CAD build for the part. Positions are in the model's coordinates, mm. A direction names the side the tool comes from. Give positions to 0.01 mm unless a question says otherwise; leave off trailing zeros. Order: outer loops, then holes, each group sorted by start corner. A loop starts at its lowest first (then second) coordinate and runs counter-clockwise, first axis right, second up.
from build123d import *

# Parameters (mm, degrees)
F0_W      = 45
F0_H      = 30
F1_DEPTH  = 3
F2_R      = 5
F3_DEPTH  = 1
F4_R      = 2.5
F5_DEPTH  = 2
F6_W      = 10
F6_H      = 30
F7_DEPTH  = 80
F9_DEPTH  = 2.5
F10_R     = 8.5
F11_DEPTH = 10
F12_R     = 10
F13_R     = 10
F14_R     = 5
F15_R     = 5


with BuildPart() as f1:
    # F0 (on Top) → F1 (new body)
    with BuildSketch(Plane.XY):
        Rectangle(F0_W, F0_H)
    extrude(amount=F1_DEPTH)

    # F2 (on face) → F3 (cut)
    with BuildSketch(Plane.XY.offset(3)):
        with Locations((-11.25, 0)):
            Circle(F2_R)
    extrude(amount=-F3_DEPTH, mode=Mode.SUBTRACT)

    # F4 (on face) → F5 (cut, through all)
    with BuildSketch(Plane.XY.offset(2)):
        with Locations((-11.25, 0)):
            Circle(F4_R)
    extrude(amount=-F5_DEPTH, mode=Mode.SUBTRACT)

    # F6 (on face) → F7 (join)
    with BuildSketch(Plane.XY.offset(3)):
        with Locations((17.5, 0)):
            Rectangle(F6_W, F6_H)
    extrude(amount=F7_DEPTH)

    # F8 (on Front) → F9 (join, symmetric)
    with BuildSketch(Plane.XZ):
        Polygon((12.5, 38), (-2.5, 3), (12.5, 3), align=None)
    extrude(amount=F9_DEPTH, both=True)

    # F10 (on face) → F11 (cut, through all)
    with BuildSketch(Plane.YZ.offset(22.5)):
        with Locations((0, 68.5)):
            Circle(F10_R)
    extrude(amount=-F11_DEPTH, mode=Mode.SUBTRACT)

    # F12
    f12_edges = [f1.edges().sort_by_distance(p)[0] for p in [
        (17.5, 15, 83),
    ]]
    fillet(f12_edges, radius=F12_R)

    # F13
    f13_edges = [f1.edges().sort_by_distance(p)[0] for p in [
        (17.5, -15, 83),
    ]]
    fillet(f13_edges, radius=F13_R)

    # F14
    f14_edges = [f1.edges().sort_by_distance(p)[0] for p in [
        (-22.5, 15, 1.5),
    ]]
    fillet(f14_edges, radius=F14_R)

    # F15
    f15_edges = [f1.edges().sort_by_distance(p)[0] for p in [
        (-22.5, -15, 1.5),
    ]]
    fillet(f15_edges, radius=F15_R)


solid = f1.part
1. Saw through at D-D on x = 5. Give the cut face in (y, z), plus the area to 4 significant figures.
2. Saw through at A-A on x = -11.25. Give the cut face in (y, z), plus the area to 3 significant figures.
3. Saw through at B-B on y = 0. Give the cut face in (x, z).
4. Saw through at C-C on z = 68.5. Give the cut face in (x, y).
5. 3-axis set-ups, long thin cutter, end or side, ignore diameter. For faces 4 (the flat face through (16, 15, 34)), 5 (the flat face through (-14, -1, 2)), 6 (the flat face through (12.5, 0, 42)), 7 (the flat face through (8, 2.5, 13)): which of +Z, -Z, +X, -X, +Y, -Y reach the whole face in a straight line?
6. Mould opens along Y. For faces 1 (the cylindrical face through (-13.748, 0.11, 1.014)), 2 (the cylindrical face through (-21, 13.57, 1.52)), 3 (the flat face through (16, -15, 34)) say: released by +Y, released by -Y, zero draft, split by the parting line, or undercut.
7. Pin check, flat tips, straight feed: P1, Ø4, axis at y = 3.5, z = 23, coming from the -X side; P2, Ø1.5, axis at x = -4, y = 7, coming from the +Z side; P3, Ø12, axis at y = -1.5, z = 47, coming from the -X side. Stop position of each tip, or through.
8. Wall check: line 1 (Z direction, x = 19, y = 0); line 2 (Y direction, x = -11.25, z = 2.25); line 3 (X direction, y = 4, z = 8). Give the ranges that are in metal, low to high.
Reported:
1. outline: (-15, 0) - (15, 0) - (15, 3) - (2.5, 3) - (2.5, 20.5) - (-2.5, 20.5) - (-2.5, 3) - (-15, 3) - close
1. area: 177.5 mm2
2. outline: (-15, 0) - (-2.5, 0) - (-2.5, 2) - (-5, 2) - (-5, 3) - (-15, 3) - close; (2.5, 0) - (15, 0) - (15, 3) - (5, 3) - (5, 2) - (2.5, 2) - close
2. area: 70.0 mm2
3. outline: (-22.5, 0) - (-13.75, 0) - (-13.75, 2) - (-16.25, 2) - (-16.25, 3) - (-22.5, 3) - close; (-8.75, 0) - (22.5, 0) - (22.5, 60) - (12.5, 60) - (12.5, 38) - (-2.5, 3) - (-6.25, 3) - (-6.25, 2) - (-8.75, 2) - close; (12.5, 77) - (22.5, 77) - (22.5, 83) - (12.5, 83) - close
4. outline: (12.5, -15) - (22.5, -15) - (22.5, -8.5) - (12.5, -8.5) - close; (12.5, 8.5) - (22.5, 8.5) - (22.5, 15) - (12.5, 15) - close
5. face 4: +Z, -Z, +X, -X, +Y
5. face 5: +Z
5. face 6: +Z, -X
5. face 7: +Z, -X, +Y
6. face 1: undercut
6. face 2: released by +Y
6. face 3: released by -Y
7. P1: stops at x = 5.33
7. P2: stops at z = 3
7. P3: stops at x = 12.5
8. line 1: z = 0 to 60, 77 to 83
8. line 2: y = -15 to -5, 5 to 15
8. line 3: x = 12.5 to 22.5
